from build123d import *

# Parameters (mm, degrees)
F3_D           = 10.71626
F3_DEPTH       = 191.008
F3_CSINK_D     = 15.875
F3_CSINK_ANGLE = 90
F5_D           = 10.71626
F5_DEPTH       = 241.808
F6_R           = 0.508


with BuildPart() as f1:
    # F0 (on Right) → F1 (revolve)
    with BuildSketch(Plane.YZ):
        Polygon((0, 28.2575), (0, 0), (279.4, 0), (279.4, 15.875), (88.646, 15.875), (35.56, 28.2575), align=None)
    revolve(axis=Axis((0, 139.7, 0), (0, 1, 0)))

    # F3
    with Locations(Plane(origin=(0, 279.4, 0), x_dir=(-1, 0, 0), z_dir=(0, 1, 0))):
        with Locations((0, 0)):
            CounterSinkHole(F3_D / 2, F3_CSINK_D / 2, depth=F3_DEPTH, counter_sink_angle=F3_CSINK_ANGLE)

    # F5
    with Locations(Plane.XZ):
        with Locations((0, 0)):
            Hole(F5_D / 2, depth=F5_DEPTH)

    # F6
    f6_edges = [f1.edges().sort_by_distance(p)[0] for p in [
        (0, 0, -28.2575),
        (0, 35.56, -28.2575),
        (0, 88.646, -15.875),
        (0, 279.4, -15.875),
    ]]
    fillet(f6_edges, radius=F6_R)


solid = f1.part
Source: CAD feature listing. Evaluate the final solid. Frame: model axes, mm. Round coordinates to 2 decimals unless told otherwise and drop trailing zeros. Order: outer loops, then holes, each group sorted by start corner. A loop starts at its lowest first (then second) coordinate and runs counter-clockwise, first axis right, second up. Notation, with made-up numbers: (-10.5, 86.5) - (19.5, 86.5) arc R23 ccw to (19.5, 117.5) - close; hole circle Ø7 at (77.25, 42.5). An arc over 180 degrees is marked (long way). Use a Markdown table: item, result. Add a question column.
1. First-contact query: pin 1 (6 mm diameter, centred on x = -19, y = 189, fed in from -Z) (3 decimals); pin 2 (1 mm diameter, centred on x = -10.5, y = 164, fed in from +Z); pin 3 (1 mm diameter, centred on x = 18, y = 52.5, fed in from +Z); pin 4 (5 mm diameter, centred on x = 0, y = 179.5, fed in from +Z) (3 decimals). Flat tips, straight axial feed; report the tip coordinate or a pass-through.
2. Section query B-B (y = 55). Return the cut outline in (x, z), then the cut area to 3 significant figures.
3. Section query A-A (y = 229). Return the cut outline in (x, z) (3 decimals).
4. Line query: probe 1 along X at (y, z) = (256, 0) (3 decimals); probe 2 along X at (y, z) = (25, 0). Output: solid intervals per line, ascending.
5. Mould query, pull axis Z, two halves, no side actions, for faces 1 (the conical face through (-0.71, 276.95, 5.44)), 2 (the cylindrical face through (4.77, 182.47, 15.14)), 3 (the flat face through (-7, 279.4, -7)). Classes: +Z half, -Z half, draft (parallel to the pull), parting line (faces both ways), or undercut.
Derived:
| question | item | result |
|---|---|---|
| 1 | pin 1 | through |
| 1 | pin 2 | z = 12.33 |
| 1 | pin 3 | z = 16.89 |
| 1 | pin 4 | z = 15.875 |
| 2 | outline | circle Ø47.45 at (0, 0); hole circle Ø10.72 at (0, 0) |
| 2 | area | 1,680 mm2 |
| 3 | outline | circle Ø31.75 at (0, 0); hole circle Ø10.716 at (0, 0) |
| 4 | probe 1 | -15.875 to -5.358, 5.358 to 15.875 |
| 4 | probe 2 | -28.26 to -5.36, 5.36 to 28.26 |
| 5 | face 1 | undercut |
| 5 | face 2 | parting line |
| 5 | face 3 | draft |
